Job drawing, mm, ordinate dimensions from the low corner. One solid piece. A direction names the side the tool comes from. Give positions to 0.01 mm unless a question says otherwise; leave off trailing zeros. Loops run counter-clockwise (first coordinate to the right, second up) from the corner with the lowest first, then second, coordinate; pieces in that order, holes last. Notation, with made-up numbers: M 88,62.5 L 102,62.5 A33 ccw 102,100.5 Z; hole C 12.5,6.5 d10. An arc over 180 degrees is marked long. Put each result on its own line as item: value.
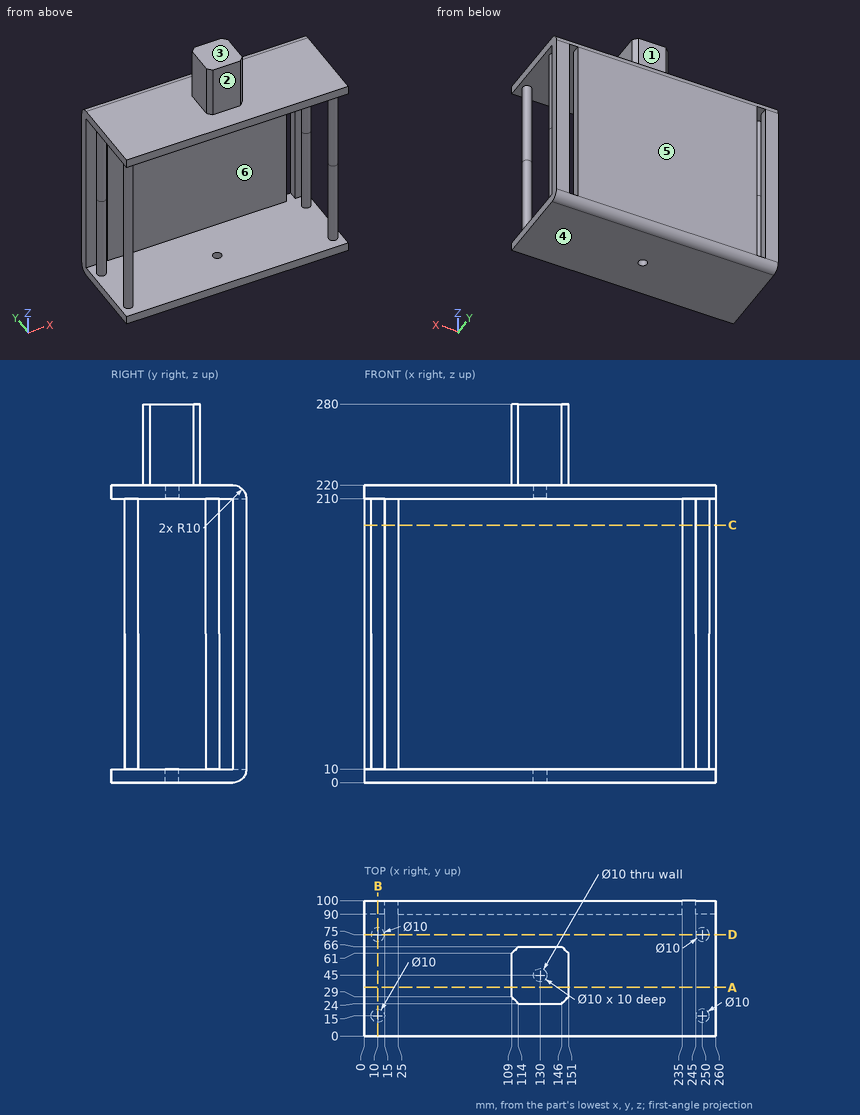
Q1. Slice it at A-A (y = 36). List the corners of the cut face in (x, z), and give its area (3 significant figures).
Here are the results:
outline: M 0,0 L 260,0 L 260,10 L 0,10 Z; M 0,210 L 260,210 L 260,220 L 151,220 L 151,280 L 109,280 L 109,220 L 0,220 Z
area: 7,720 mm²
Q2. Probe line 1 (Z direction, x = 212.5, y = 73.5); line 2 (Z direction, x = 115, y = 45.5); line 3 (Y direction, x = 53, z = 51). List the from-to ranges inside material, lowest first. Write a range as from..to.
Here are the results:
line 1: 0..10, 210..220
line 2: 0..10, 210..280
line 3: 90..100
Q3. Slice it at C-C (z = 190.5). List the corners of the cut face in (x, y).
Here are the results:
outline: M 0,90 L 15,90 L 15,100 L 0,100 Z; C 10,15 d10; C 10,75 d10; M 25,90 L 235,90 L 235,100 L 25,100 Z; C 250,15 d10; C 250,75 d10; M 245,90 L 260,90 L 260,100 L 245,100 Z
Q4. Mould opens along Z. For the marked faces 3, 4, 5 and 6 say: pulls with the +Z half, pulls with the -Z half, needs draft (parallel to the pull), parting line crosses it, or undercut.
Here are the results:
face 3: pulls with the +Z half
face 4: pulls with the -Z half
face 5: needs draft
face 6: undercut
Q5. Drop flat-ended pins along their axis: pin 1 Ø12 at (x, z) = (7.5, 160) entering from -Y; pin 2 Ø16 at (x, z) = (129.5, 256) entering from +Y; pin 3 Ø8 at (x, y) = (130, 45) entering from -Z; pin 4 Ø3 at (y, z) = (96, 147.5) entering from -X. Give the stop position or say it passes through.
Here are the results:
pin 1: y = 10
pin 2: y = 66
pin 3: z = 220
pin 4: x = 0
Q6. Tool access for the marked faces 1 and 2: list every direction of +Z, -Z, +X, -X, +Y, -Y with a clear straight run to the whole face (end or side of a thin tool).
Here are the results:
face 1: +Z, +X, -X, +Y
face 2: +Z, +X, -X, -Y
Q7. Slice it at D-D (y = 75). List the corners of the cut face in (x, z).
Here are the results:
outline: M 0,0 L 260,0 L 260,10 L 255,10 L 255,210 L 260,210 L 260,220 L 0,220 L 0,210 L 5,210 L 5,10 L 0,10 Z; hole M 15,10 L 245,10 L 245,210 L 15,210 Z
Q8. Slice it at B-B (x = 10). List the corners of the cut face in (y, z), and give its area (3 significant figures).
Here are the results:
outline: M 0,0 L 90,0 A10 ccw 100,10 L 100,210 A10 ccw 90,220 L 0,220 L 0,210 L 10,210 L 10,10 L 0,10 Z; hole M 20,10 L 70,10 L 70,210 L 20,210 Z; hole M 80,10 L 90,10 L 90,210 L 80,210 Z
area: 7,960 mm²
